The figure shows three views and two pictorial views of one solid part (mm, origin at its lowest corner). Answer the questions. A direction names the side the tool comes from. Give positions to 0.01 mm unless a question says otherwise; leave off trailing zeros. Loops run counter-clockwise (first coordinate to the right, second up) from the corner with the lowest first, then second, coordinate; pieces in that order, holes last. Notation, with made-up numbers: (-6.5, 41.5) - (0.5, 41.5) arc R19 cw to (0.5, 71.5) - close; hole circle Ø5 at (58, -29.5). An arc over 180 degrees is marked (long way). One line per question, with ' | ' between items.
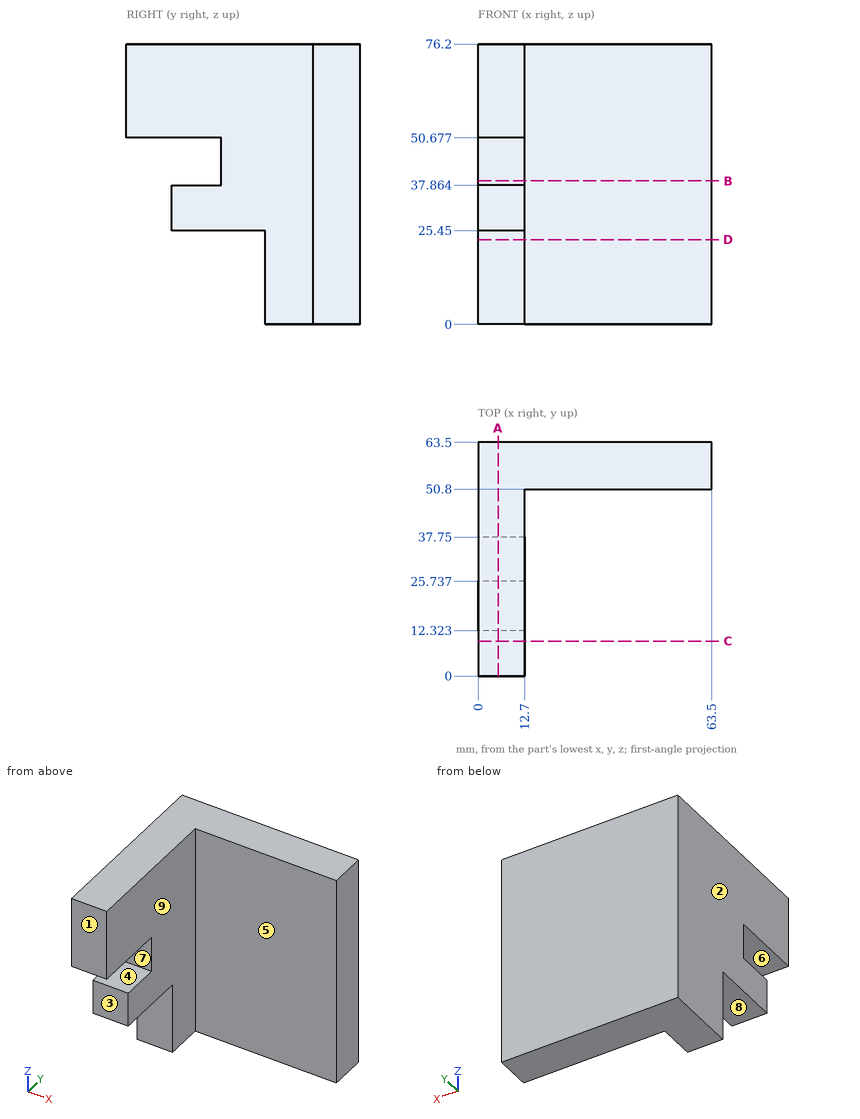
1. Find section B-B on z = 39. Write down the section's boundary in (x, y), then the cut area to 3 significant figures.
Evaluation:
outline: (0, 25.74) - (12.7, 25.74) - (12.7, 50.8) - (63.5, 50.8) - (63.5, 63.5) - (0, 63.5) - close | area: 1,120 mm2
2. Find section D-D on z = 23. Write down the section's boundary in (x, y).
Evaluation:
outline: (0, 37.75) - (12.7, 37.75) - (12.7, 50.8) - (63.5, 50.8) - (63.5, 63.5) - (0, 63.5) - close
3. Find section A-A on x = 5.5. Write down the section's boundary in (y, z), then the cut area to 4 significant figures.
Evaluation:
outline: (0, 50.68) - (25.74, 50.68) - (25.74, 37.86) - (12.32, 37.86) - (12.32, 25.45) - (37.75, 25.45) - (37.75, 0) - (63.5, 0) - (63.5, 76.2) - (0, 76.2) - close | area: 3,395 mm2
4. Determine the mould class of the marked faces 6, 7, 8 and 9 for opening direction Z: +Z half, -Z half, draft (parallel to the pull), parting line (faces both ways), or undercut.
Evaluation:
face 6: undercut | face 7: undercut | face 8: -Z half | face 9: draft
5. Which of the six approach directions +Z, -Z, +X, -X, +Y, -Y give full straight-line access (tool end or side, diameter ignored) to the marked faces 1, 2, 3, 4 and 5?
Evaluation:
face 1: +Z, -Z, +X, -X, -Y | face 2: +Z, -Z, -X, +Y, -Y | face 3: -Z, +X, -X, -Y | face 4: +X, -X, -Y | face 5: +Z, -Z, +X, -Y
6. Flat-ended cylindrical pins translate along their axes: pin 1 (15 mm diameter, centred on x = 47, z = 43.5, fed in from -Y); pin 2 (6.5 mm diameter, centred on x = 3.5, y = 12, fed in from -Z); pin 3 (6.5 mm diameter, centred on x = 8.5, z = 45.5, fed in from -Y); pin 4 (1.5 mm diameter, centred on x = 13.5, y = 7.5, fed in from +Z). Find the tip coordinate at first contact, or state that the pin passes through.
Evaluation:
pin 1: y = 50.8 | pin 2: z = 25.45 | pin 3: y = 25.74 | pin 4: through
7. Consider L1, parallel to Z at x = 7, y = 19; L2, parallel to Y at x = 38.5, z = 50.5; L3, parallel to X at y = 12.5, z = 58.5. Determine where each line is inside the solid, lowest interval first.
Evaluation:
L1: 25.45 to 37.86, 50.68 to 76.2 | L2: 50.8 to 63.5 | L3: 0 to 12.7
8. Find section C-C on y = 9.5. Write down the section's boundary in (x, z), then the cut area to 3 significant figures.
Evaluation:
outline: (0, 50.68) - (12.7, 50.68) - (12.7, 76.2) - (0, 76.2) - close | area: 324 mm2
